Work out the finished part from the listing and answer in its coordinate system (mm). Face numbers are marked on the shaded views. Give positions to 0.01 mm unless a question says otherwise; leave off trailing zeros. Order: outer loops, then holes, each group sorted by start corner. A loop starts at its lowest first (then second) coordinate and runs counter-clockwise, first axis right, second up. Notation, with made-up numbers: (87.5, -32) -> (133.5, -32) arc R28 ccw to (133.5, -13) -> close; hole circle Ø10 at (11, 46.5). An arc over 180 degrees is marked (long way). Answer as CSV lines item,"result". Start each with the question number.
1. For a pull along Z with two mould halves and no side action, classify the marked faces 1, 2 and 3 as released by +Z, released by -Z, zero draft, split by the parting line, or undercut.
2. A cutting plane is placed at D-D (x = -0.95). Give the vertices of the cut face in (y, z).
3. Find the intervals of material crossed by L1, parallel to Y at x = 0.5, z = -5.75; L2, parallel to X at y = 5, z = -9.75; L3, parallel to Y at x = -0.5, z = -8.5, in increasing order.
4. A cutting plane is placed at A-A (x = 1.1). Give the vertices of the cut face in (y, z), then the cut area to 3 significant figures.
5. A cutting plane is placed at B-B (y = 25.45). Give the vertices of the cut face in (x, z), then the cut area to 4 significant figures.
6. A cutting plane is placed at C-C (y = 5). Give the vertices of the cut face in (x, z).
from build123d import *

# Parameters (mm, degrees)
SKETCH1_W           = 4.5
SKETCH1_H           = 15
BOSS_EXTRUDE1_DEPTH = 31
SKETCH2_R           = 3.55
CUT_EXTRUDE1_DEPTH  = 20
SKETCH3_R           = 1.5
CUT_EXTRUDE2_DEPTH  = 20
SKETCH4_R           = 1.5
CUT_EXTRUDE3_DEPTH  = 20
FILLET1_R           = 3
FILLET2_R           = 3


with BuildPart() as part:
    # Sketch1 → Boss-Extrude1 (new body)
    with BuildSketch(Plane(origin=(0, 0, 0), x_dir=(1, 0, 0), z_dir=(0, 1, 0))):
        with Locations((-0.136363636, 6.163636364)):
            Rectangle(SKETCH1_W, SKETCH1_H)
    extrude(amount=BOSS_EXTRUDE1_DEPTH)

    # Sketch2 → Cut-Extrude1 (cut)
    with BuildSketch(Plane(origin=(2.113636364, 0, 0), x_dir=(0, 0, -1), z_dir=(1, 0, 0))):
        with Locations((6.163636364, 25.45)):
            Circle(SKETCH2_R)
    extrude(amount=-CUT_EXTRUDE1_DEPTH, mode=Mode.SUBTRACT)

    # Sketch3 → Cut-Extrude2 (cut)
    with BuildSketch(Plane.ZY.offset(2.386363636)):
        with Locations((-6.163636364, 5)):
            Circle(SKETCH3_R)
    extrude(amount=-CUT_EXTRUDE2_DEPTH, mode=Mode.SUBTRACT)

    # Sketch4 → Cut-Extrude3 (cut)
    with BuildSketch(Plane(origin=(0, 0, -13.663636364), x_dir=(-1, 0, 0), z_dir=(0, 0, -1))):
        with Locations((0, 5)):
            Circle(SKETCH4_R)
    extrude(amount=-CUT_EXTRUDE3_DEPTH, mode=Mode.SUBTRACT)

    # Fillet1
    fillet1_edges = [part.edges().sort_by_distance(p)[0] for p in [
        (-0.136363636, 31, 1.336363636),
    ]]
    fillet(fillet1_edges, radius=FILLET1_R)

    # Fillet2
    fillet2_edges = [part.edges().sort_by_distance(p)[0] for p in [
        (-0.136363636, 31, -13.663636364),
    ]]
    fillet(fillet2_edges, radius=FILLET2_R)


solid = part.part
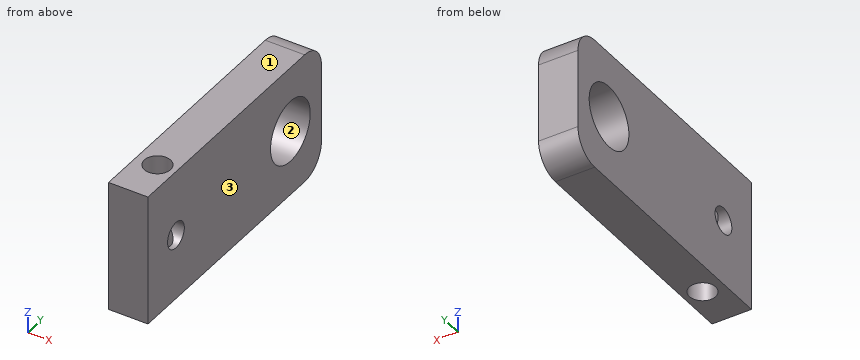
Answer sheet:
1,face 1,"released by +Z"
1,face 2,"undercut"
1,face 3,"zero draft"
2,outline,"(0, -13.66) -> (3.84, -13.66) -> (3.84, -7.11) arc R1.5 cw to (3.84, -5.21) -> (3.84, 1.34) -> (0, 1.34) -> close; (6.16, -13.66) -> (28, -13.66) arc R3 ccw to (31, -10.66) -> (31, -1.66) arc R3 ccw to (28, 1.34) -> (6.16, 1.34) -> (6.16, -5.21) arc R1.5 cw to (6.16, -7.11) -> close; hole circle Ø7.1 at (25.45, -6.16)"
3,L1,"y = 0 to 3.56, 6.44 to 21.92, 28.98 to 31"
3,L2,"x = -2.39 to -1.5, 1.5 to 2.11"
3,L3,"y = 0 to 3.59, 6.41 to 22.78, 28.12 to 31"
4,outline,"(0, -13.66) -> (3.98, -13.66) -> (3.98, -7.26) arc R1.5 cw to (3.98, -5.06) -> (3.98, 1.34) -> (0, 1.34) -> close; (6.02, -13.66) -> (28, -13.66) arc R3 ccw to (31, -10.66) -> (31, -1.66) arc R3 ccw to (28, 1.34) -> (6.02, 1.34) -> (6.02, -5.06) arc R1.5 cw to (6.02, -7.26) -> close; hole circle Ø7.1 at (25.45, -6.16)"
4,area,"389 mm^2"
5,outline,"(-2.39, -13.66) -> (2.11, -13.66) -> (2.11, -9.71) -> (-2.39, -9.71) -> close; (-2.39, -2.61) -> (2.11, -2.61) -> (2.11, 1.34) -> (-2.39, 1.34) -> close"
5,area,"35.55 mm^2"
6,outline,"(-2.39, -13.66) -> (-1.5, -13.66) -> (-1.5, -7.66) -> (-2.39, -7.66) -> close; (-2.39, -4.66) -> (-1.5, -4.66) -> (-1.5, 1.34) -> (-2.39, 1.34) -> close; (1.5, -13.66) -> (2.11, -13.66) -> (2.11, -7.66) -> (1.5, -7.66) -> close; (1.5, -4.66) -> (2.11, -4.66) -> (2.11, 1.34) -> (1.5, 1.34) -> close"
